```python
from build123d import *

# Parameters (mm, degrees)
MODEL_R                 = 5.602685567
MODEL_R_2               = 2
MODEL_W                 = 10
MODEL_H                 = 3
SALIENTE_EXTRUIR1_DEPTH = 3


with BuildPart() as part:
    # Model → Saliente-Extruir1 (new body)
    with BuildSketch(Plane.XY):
        with BuildLine():
            Line((40.656841206, 68.2), (-1.7, 68.2))
            Line((-1.7, 68.2), (-29.984726632, 48.394821196))
            ThreePointArc((-29.984726632, 48.394821196), (-31.349079816, 47.721996664), (-32.852608814, 47.490581417))
            Line((-32.852608814, 47.490581417), (-42.689839841, 47.490581417))
            ThreePointArc((-42.689839841, 47.490581417), (-46.225125286, 46.026363766), (-47.689839791, 42.491284145))
            Line((-47.689839791, 42.491284145), (-47.7, -29.8))
            Line((-47.7, -29.8), (-18.946904924, -29.8))
            Line((-18.946904924, -29.8), (62.3, -29.8))
            Line((62.3, -29.8), (69.836645163, -29.8))
            Line((69.836645163, -29.8), (73.3, -29.8))
            Line((73.3, -29.8), (94.3, -29.8))
            Line((94.3, -29.8), (94.289839791, 42.491284145))
            ThreePointArc((94.289839791, 42.491284145), (92.825125286, 46.026363766), (89.289839841, 47.490581417))
            Line((89.289839841, 47.490581417), (79.452608814, 47.490581417))
            ThreePointArc((79.452608814, 47.490581417), (77.949079816, 47.721996664), (76.584726632, 48.394821196))
            Line((76.584726632, 48.394821196), (48.3, 68.2))
            Line((48.3, 68.2), (40.656841206, 68.2))
        make_face()
        with Locations((-20.7, 22.2)):
            Circle(MODEL_R, mode=Mode.SUBTRACT)
        with Locations((67.3, 22.2)):
            Circle(MODEL_R, mode=Mode.SUBTRACT)
        with Locations((42.3, 61.2)):
            Circle(MODEL_R_2, mode=Mode.SUBTRACT)
        with Locations((4.3, 61.2)):
            Circle(MODEL_R_2, mode=Mode.SUBTRACT)
        with Locations((4.3, 55.2)):
            Rectangle(MODEL_W, MODEL_H, mode=Mode.SUBTRACT)
        Polygon((58.660844318, 47.809630387), (60.381573627, 50.26708652), (52.190053184, 56.002850883), (50.469323875, 53.545394751), align=None, mode=Mode.SUBTRACT)
        with Locations((42.3, 55.2)):
            Rectangle(MODEL_W, MODEL_H, mode=Mode.SUBTRACT)
        Polygon((-12.060844318, 47.809630387), (-13.781573627, 50.26708652), (-5.590053184, 56.002850883), (-3.869323875, 53.545394751), align=None, mode=Mode.SUBTRACT)
        Polygon((-34.997101558, 31.749490169), (-36.717830867, 34.206946302), (-44.90935131, 28.471181939), (-43.188622001, 26.013725806), align=None, mode=Mode.SUBTRACT)
        Polygon((81.597101558, 31.749490169), (83.317830867, 34.206946302), (91.50935131, 28.471181939), (89.788622001, 26.013725806), align=None, mode=Mode.SUBTRACT)
    extrude(amount=SALIENTE_EXTRUIR1_DEPTH)


solid = part.part
```
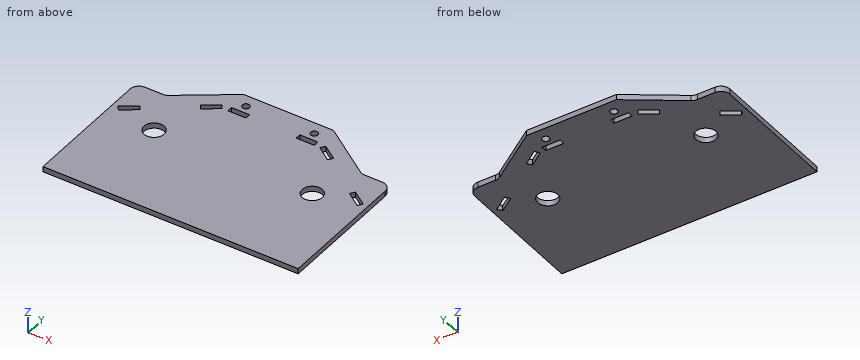
Geometry: final body of the model. Coordinates: model frame, mm. Round coordinates to 2 decimals unless told otherwise and drop trailing zeros. Write each loop counter-clockwise with the first axis right and the second up, starting at its lowest first coordinate (ties: lowest second). Pieces come first, ordered by that corner, then holes.
Item 1: Pin query (flat end, axial travel): P1, Ø4.5, axis at x = 4.3, y = 61.2, coming from the +Z side; P2, Ø0.9, axis at x = -38.5, z = 1.5, coming from the +Y side; P3, Ø1.5, axis at y = 54.5, z = 2, coming from the +X side; P4, Ø1.5, axis at y = 54.5, z = 2, coming from the -X side. Return the tip coordinate at first contact, or that it passes through.
Item 2: Section query D-D (x = 57). Return loops of the section in (y, z), plus the area to 3 significant figures.
Item 3: Section query C-C (z = 1.2). Give the number of separate pieces and of enclosed holes in the cut face, plus the area to 3 significant figures.
Item 4: Section query A-A (x = 42.3). Return loops of the section in (y, z).
Item 5: Material intervals for L1, parallel to Y at x = 4.3, z = 1.2; L2, parallel to X at y = 62, z = 0.5; L3, parallel to X at y = 51.5, z = 1.35, sorted ascending.
Item 6: Section query B-B (y = 61.2). Return loops of the section in (x, z), plus the area to 3 significant figures.
Completed:
1. P1: stops at z = 3
1. P2: stops at y = 47.49
1. P3: stops at x = 68.94
1. P4: stops at x = -22.34
2. outline: (-29.8, 0) - (48.97, 0) - (48.97, 3) - (-29.8, 3) - close; (52.63, 0) - (62.11, 0) - (62.11, 3) - (52.63, 3) - close
2. area: 265 mm2
3. separate pieces: 1
3. enclosed holes: 10
3. area: 12,200 mm2
4. outline: (-29.8, 0) - (53.7, 0) - (53.7, 3) - (-29.8, 3) - close; (56.7, 0) - (59.2, 0) - (59.2, 3) - (56.7, 3) - close; (63.2, 0) - (68.2, 0) - (68.2, 3) - (63.2, 3) - close
5. L1: y = -29.8 to 53.7, 56.7 to 59.2, 63.2 to 68.2
5. L2: x = -10.55 to 2.47, 6.13 to 40.47, 44.13 to 57.15
5. L3: x = -25.55 to -12.02, -6.79 to 53.39, 58.62 to 72.15
6. outline: (-11.7, 0) - (2.3, 0) - (2.3, 3) - (-11.7, 3) - close; (6.3, 0) - (40.3, 0) - (40.3, 3) - (6.3, 3) - close; (44.3, 0) - (58.3, 0) - (58.3, 3) - (44.3, 3) - close
6. area: 186 mm2
